The listing builds one solid part. Answer for the finished solid, in the listing's coordinates (mm). Face numbers are marked on the shaded views. A direction names the side the tool comes from. Give positions to 0.01 mm unless a question says otherwise; leave off trailing zeros. Loops run counter-clockwise (first coordinate to the right, second up) from the corner with the lowest first, then second, coordinate; pieces in that order, holes last. Notation, with made-up numbers: (47.5, -32.75) - (89.5, -32.75) arc R22 cw to (89.5, -16.75) - close; hole circle Ø6 at (74, 26). An arc over 180 degrees is marked (long way). One line per item, written item: value. Start each with the question number.
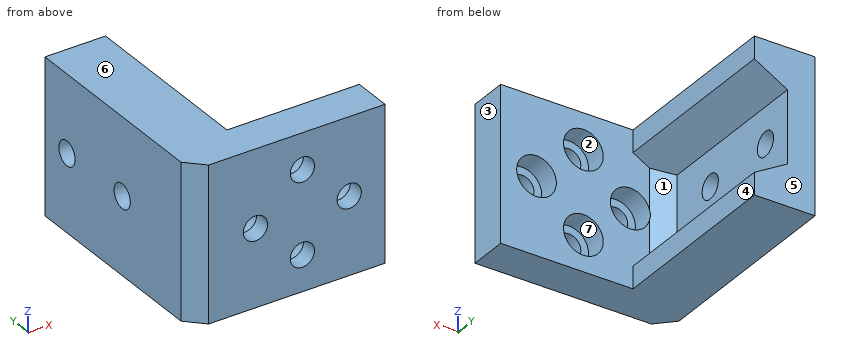
Autodesk Inventor part; units mm, degrees
ref_plane "YZ Plane" through (0, 0, 0) normal (1, 0, 0) x (0, 1, 0)
ref_plane "XZ Plane" through (0, 0, 0) normal (0, 1, 0) x (-1, 0, 0)
ref_plane "XY Plane" through (0, 0, 0) normal (0, 0, 1) x (1, 0, 0)
sketch "Sketch1" plane through (0, 0, 0) normal (0, 0, 1) x (1, 0, 0)
  line L0 (35, 0) -> (0, 0)
  line L1 (0, 0) -> (0, 40)
  line L2 (0, 40) -> (5, 40)
  line L3 (5, 40) -> (5, 7)
  line L4 (5, 7) -> (35, 7)
  line L5 (35, 7) -> (35, 0)
  line L6 (-7, 0) -> (42, 0)
  line L7 (0, -8) -> (0, 48)
  dimension "d0" = 7
  dimension "d1" = 5
  dimension "d2" = 40
  dimension "d3" = 30
extrude "Extrusion1" add sketch "Sketch1" along normal mid plane 28
sketch "Sketch2" plane through (5, 7, 14) normal (0, 1, 0) x (1, 0, 0)
  circle A0 centre (15, 21.5) radius 2.2
  circle A1 centre (23.5, 14) radius 2.2
  circle A2 centre (15, 6.5) radius 2.2
  circle A3 centre (6.5, 14) radius 2.2
  point P0 (-5, 14)
extrude "Extrusion2" cut sketch "Sketch2" against normal through all
sketch "Sketch3" plane through (5, 7, 14) normal (0, 1, 0) x (1, 0, 0)
  circle A0 centre (15, 6.5) radius 2.2
  circle A1 centre (15, 21.5) radius 2.2
  circle A2 centre (23.5, 14) radius 2.2
  circle A3 centre (6.5, 14) radius 2.2
  line L0 (0, 28) -> (0, 0)
  line L1 (30, 0) -> (0, 0)
  line L2 (30, 28) -> (30, 0)
  line L3 (0, 28) -> (30, 28)
  circle A4 centre (6.5, 14) radius 3.6
  circle A5 centre (15, 21.5) radius 3.6
  circle A6 centre (23.5, 14) radius 2.2
  circle A7 centre (23.5, 14) radius 3.6
  circle A8 centre (15, 6.5) radius 3.6
  point P0 (-5, 14)
  dimension "d8" = 7.2
extrude "Extrusion3" cut sketch "Sketch3" against normal blind 4 contours A4 | A5 | A7 | A8
chamfer "Chamfer1" distance 3 angle 45 1 edges at (5, 7, 0)
sketch "Sketch4" plane through (5, 40, 14) normal (1, 0, 0) x (0, 0, -1)
  line L0 (28, 0) -> (0, 0)
  line L1 (14, 0) -> (14, -21)
  circle A0 centre (14, -21) radius 2.2
  circle A1 centre (14, -6) radius 2.2
  point P0 (14, -40)
  dimension "d14" = 4.4
  dimension "d15" = 15
  dimension "d16" = 6
extrude "Extrusion4" cut sketch "Sketch4" against normal through all
chamfer "Chamfer2" distance 3 angle 45 1 edges at (0, 0, 0)
sketch "Sketch5" plane through (0, 40, 14) normal (0, 1, 0) x (1, 0, 0)
  line L0 (5, 28) -> (5, 0)
  line L1 (5, 28) -> (11, 28)
  line L2 (35, 28) -> (3, 28)
  line L3 (11, 24) -> (5, 20.5359)
  line L4 (11, 28) -> (11, 24)
  point P0 (0, 14)
  dimension "d22" = 60
  dimension "d23" = 6
  dimension "d24" = 4
extrude "Extrusion5" add sketch "Sketch5" against normal up to surface (33 mm away)
mirror "Mirror1" about plane through (0, 0, 0) normal (0, 0, 1) of "Extrusion5"
sketch "Sketch6" plane through (0, 40, -14) normal (-1, 0, 0) x (0, 0, 1)
  line L0 (0, 0) -> (28, 0)
  line L1 (8, 0) -> (20, 0)
  line L2 (20, 0) -> (20, -26)
  line L3 (20, -26) -> (8, -26)
  line L4 (8, -26) -> (8, 0)
  circle A0 centre (14, -21) radius 2.2
  point P0 (14, -40)
  point P1 (14, 0)
  dimension "d27" = 12
  dimension "d28" = 5
split_face "Split1"
properties part number "Test Mount"
1. For the marked faces 1, 2, 3 and 4, determine the directions among +Z, -Z, +X, -X, +Y, -Y from which every point of the face is accessible in a straight line to the end or side of a thin tool.
2. Find the intervals of material crossed by L1, parallel to Z at x = 20, y = 1.2; L2, parallel to Z at x = 20, y = 4.9; L3, parallel to X at y = 3.8, z = -7.5, in increasing order. Write a range as [from, to].
3. Determine the mould class of the marked faces 5, 6 and 7 for opening direction Z: released by +Z, released by -Z, zero draft, split by the parting line, or undercut.
4. A cutting plane is placed at C-C (z = 0). Give the number of separate pieces and of enclosed holes in the cut face, plus the area to 3 significant figures.
5. Flat-ended cylindrical pins translate along their axes: pin 1 (3 mm diameter, centred on y = 17.5, z = 12, fed in from +X); pin 2 (8 mm diameter, centred on x = 20, z = 9, fed in from +Y); pin 3 (1.5 mm diameter, centred on y = 18.5, z = -1.5, fed in from +X). Find the tip coordinate at first contact, or state that the pin passes through.
6. A cutting plane is placed at B-B (y = 19). Determine the outline of the cut face in (x, z), plus the area to 3 significant figures.
7. A cutting plane is placed at D-D (z = -8.75). Determine the outline of the cut face in (x, y).
8. A cutting plane is placed at A-A (x = 20). Determine the outline of the cut face in (y, z).
Results below:
1. face 1: +X, +Y
1. face 2: +Y
1. face 3: +Z, -Z, +X, +Y, -Y
1. face 4: +Z, -Z, +X, +Y
2. L1: z = [-14, -9.7], [-5.3, 5.3], [9.7, 14]
2. L2: z = [-14, -11.1], [-3.9, 3.9], [11.1, 14]
2. L3: x = [0, 16.4], [23.6, 35]
3. face 5: zero draft
3. face 6: released by +Z
3. face 7: undercut
4. separate pieces: 5
4. enclosed holes: 0
4. area: 282 mm^2
5. pin 1: stops at x = 11
5. pin 2: stops at y = 7
5. pin 3: stops at x = 5
6. outline: (0, -14) - (11, -14) - (11, -10) - (5, -6.54) - (5, -2.2) - (0, -2.2) - close; (0, 2.2) - (5, 2.2) - (5, 6.54) - (11, 10) - (11, 14) - (0, 14) - close
6. area: 187 mm^2
7. outline: (0, 3) - (3, 0) - (18.19, 0) - (18.19, 3) - (16.62, 3) - (16.62, 7) - (8.83, 7) - (8.83, 40) - (0, 40) - close; (21.81, 0) - (35, 0) - (35, 7) - (23.38, 7) - (23.38, 3) - (21.81, 3) - close
8. outline: (0, -14) - (7, -14) - (7, -11.1) - (3, -11.1) - (3, -9.7) - (0, -9.7) - close; (0, -5.3) - (3, -5.3) - (3, -3.9) - (7, -3.9) - (7, 3.9) - (3, 3.9) - (3, 5.3) - (0, 5.3) - close; (0, 9.7) - (3, 9.7) - (3, 11.1) - (7, 11.1) - (7, 14) - (0, 14) - close
